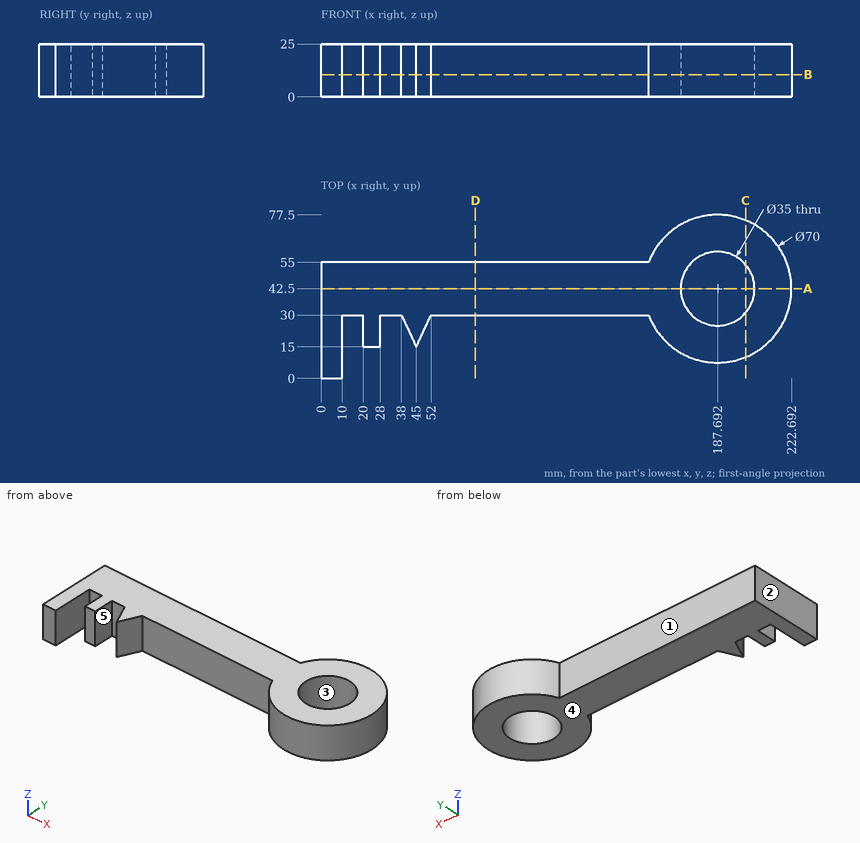
Job drawing, mm, ordinate dimensions from the low corner. One solid piece. A direction names the side the tool comes from. Give positions to 0.01 mm unless a question says otherwise; leave off trailing zeros. Loops run counter-clockwise (first coordinate to the right, second up) from the corner with the lowest first, then second, coordinate; pieces in that order, holes last. Notation, with made-up numbers: M -2,82 L 8,82 A23 cw 8,102 Z; hole C 31.5,9.25 d8. An arc over 180 degrees is marked long. Answer in a Markdown table with one row per item. Add a question column.
Item 1: Mould opens along X. For the marked faces 1, 2 and 3 say: +X half, -X half, draft (parallel to the pull), parting line (faces both ways), or undercut.
Item 2: Drop flat-ended pins along their axis: P1, Ø5, axis at x = 32.5, z = 9, coming from the -Y side; P2, Ø5, axis at y = 69, z = 15.5, coming from the +X side; P3, Ø12.5, axis at y = 12, z = 11, coming from the +X side. Give the stop position or say it passes through.
Item 3: Band-saw the part on D-D on x = 73. Give the cut face in (y, z), then the cut area to 3 significant figures.
Item 4: Band-saw the part on B-B on z = 10.5. Give the cut face in (x, y).
Item 5: Tool access for the marked faces 4 and 5: list every direction of +Z, -Z, +X, -X, +Y, -Y with a clear straight run to the whole face (end or side of a thin tool).
Item 6: Band-saw the part on A-A on y = 42.5. Give the cut face in (x, z), then the cut area to 3 significant figures.
Item 7: Band-saw the part on C-C on x = 201. Give the cut face in (y, z), then the cut area to 3 significant figures.
Item 8: Probe probe 1 along Y at (x, z) = (97.5, 11); probe 2 along X at (y, z) = (5.5, 10.5); probe 3 along X at (y, z) = (54, 20.5). List the from-to ranges inside material, lowest first.
Reply:
| question | item | result |
|---|---|---|
| 1 | face 1 | draft |
| 1 | face 2 | -X half |
| 1 | face 3 | undercut |
| 2 | P1 | stops at y = 30 |
| 2 | P2 | stops at x = 213.17 |
| 2 | P3 | stops at x = 212.93 |
| 3 | outline | M 30,0 L 55,0 L 55,25 L 30,25 Z |
| 3 | area | 625 mm^2 |
| 4 | outline | M 0,0 L 10,0 L 10,30 L 20,30 L 20,15 L 28,15 L 28,30 L 38,30 L 45,15 L 52,30 L 155,30 A35 ccw long 155,55 L 0,55 Z; hole C 187.69,42.5 d35 |
| 5 | face 4 | -Z, +X, -X, +Y, -Y |
| 5 | face 5 | +Z, -Z, -Y |
| 6 | outline | M 0,0 L 170.19,0 L 170.19,25 L 0,25 Z; M 205.19,0 L 222.69,0 L 222.69,25 L 205.19,25 Z |
| 6 | area | 4,690 mm^2 |
| 7 | outline | M 10.13,0 L 31.14,0 L 31.14,25 L 10.13,25 Z; M 53.86,0 L 74.87,0 L 74.87,25 L 53.86,25 Z |
| 7 | area | 1,050 mm^2 |
| 8 | probe 1 | y = 30 to 55 |
| 8 | probe 2 | x = 0 to 10 |
| 8 | probe 3 | x = 0 to 174.5, 200.88 to 220.75 |
